Design review of the part shown in the three views and the two pictorial views. Dimensions are in mm from the part's minimum x, y and z. A direction names the side the tool comes from. Round coordinates to 2 decimals unless told otherwise and drop trailing zeros. Order: outer loops, then holes, each group sorted by start corner. A loop starts at its lowest first (then second) coordinate and runs counter-clockwise, first axis right, second up.
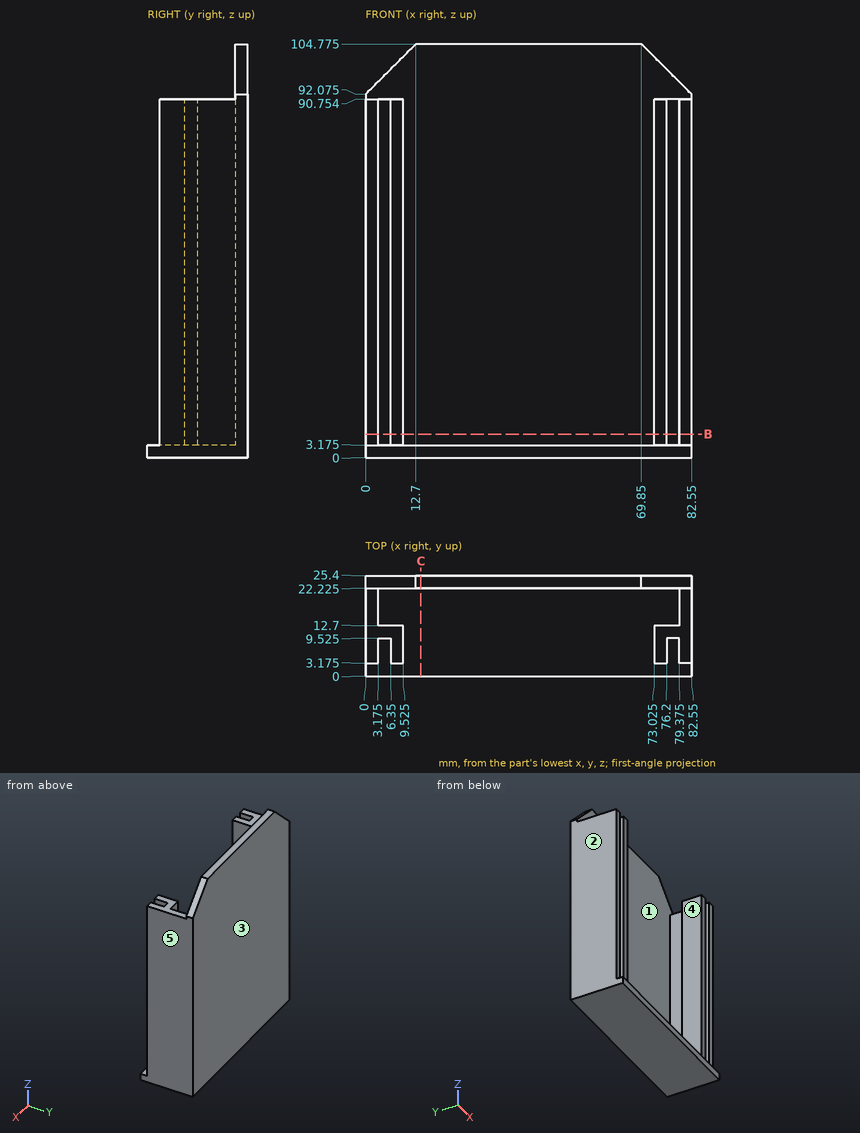
(1) For the marked faces 4 and 5, list the 3-axis set-ups (+Z, -Z, +X, -X, +Y, -Y) from which the entire face can be reached by the end or side of a thin tool; tool diameter is ignored.
Data:
face 4: +Z, -Y
face 5: +Z, -Z, +X, +Y, -Y
(2) Consider section C-C (x = 14). Write out the cut boundary in (y, z) (3 decimals).
Data:
outline: (0, 0) - (25.4, 0) - (25.4, 104.775) - (22.225, 104.775) - (22.225, 3.175) - (0, 3.175) - close
(3) Consider section B-B (z = 6). Write out the cut boundary in (x, y) (3 decimals), and give its area (3 significant figures).
Data:
outline: (0, 3.175) - (3.175, 3.175) - (3.175, 9.525) - (6.35, 9.525) - (6.35, 3.175) - (9.525, 3.175) - (9.525, 12.7) - (3.175, 12.7) - (3.175, 22.225) - (79.375, 22.225) - (79.375, 12.7) - (73.025, 12.7) - (73.025, 3.175) - (76.2, 3.175) - (76.2, 9.525) - (79.375, 9.525) - (79.375, 3.175) - (82.55, 3.175) - (82.55, 25.4) - (0, 25.4) - close
area: 464 mm2
(4) Draft analysis for pull direction X (two halves, no side actions). For the marked faces 1, 2 and 3, state which applies: pulls with the +X half, pulls with the -X half, needs draft (parallel to the pull), parting line crosses it, or undercut.
Data:
face 1: undercut
face 2: pulls with the -X half
face 3: needs draft
(5) Insertion check: pin 1 (12 mm diameter, centred on x = 45.5, y = 16, fed in from +Z) (3 decimals); pin 2 (1 mm diameter, centred on x = 7.5, z = 41.5, fed in from -Y) (3 decimals); pin 3 (10 mm diameter, centred on x = 12.5, y = 4, fed in from +Z). Each pin has a flat end and moves straight along its axis. Give the tip position at first contact, or say it passes through.
Data:
pin 1: stops at z = 3.175
pin 2: stops at y = 3.175
pin 3: stops at z = 90.75
(6) To check wall thickness, follow probe 1 along X at (y, z) = (6.5, 49) (3 decimals); probe 2 along Y at (x, z) = (4, 35) (3 decimals); probe 3 along X at (y, z) = (21, 30) (3 decimals). State the ranges of each line that lie inside material, in increasing order.
Data:
probe 1: x = 0 to 3.175, 6.35 to 9.525, 73.025 to 76.2, 79.375 to 82.55
probe 2: y = 9.525 to 12.7, 22.225 to 25.4
probe 3: x = 0 to 3.175, 79.375 to 82.55
